Work out the finished part from the listing and answer in its coordinate system (mm). A direction names the side the tool comes from. Give positions to 0.01 mm unless a question says otherwise; leave off trailing zeros. Order: outer loops, then holes, each group sorted by start corner. A loop starts at its lowest first (then second) coordinate and runs counter-clockwise, first axis right, second up. Notation, with made-up numbers: (1, -3) -> (56, -3) arc R8 ccw to (56, 9) -> close; hole circle Ø11 at (24.5, -4.75). An arc over 180 degrees is marked (long way). Answer as CSV lines item,"result". Start each with the question number.
1. For a pull along X with two mould halves and no side action, classify faces 1 (the flat face through (0, 0, 0)), 2 (the cylindrical face through (22, 30, 5)), 3 (the flat face through (14.6, 38, -7)) as released by +X, released by -X, zero draft, split by the parting line, or undercut.
2. Find the intervals of material crossed by L1, parallel to Z at x = 24, y = 29; L2, parallel to X at y = 23.5, z = -8.5; L3, parallel to Y at x = 6, z = 3.25, in increasing order.
3. A cutting plane is placed at D-D (x = 7). Give the vertices of the cut face in (y, z), then the cut area to 3 significant figures.
4. A cutting plane is placed at B-B (x = 24.25). Give the vertices of the cut face in (y, z).
5. For faces 4 (the flat face through (20.2, 14, 0)), 5 (the flat face through (4, 38, -8.85)), 6 (the flat face through (-5, 39.6, 0)), 7 (the flat face through (-23, 3.7, 0)), 8 (the flat face through (24, 31, 0)), determine the directions among +Z, -Z, +X, -X, +Y, -Y from which every point of the face is accessible in a straight line to the end or side of a thin tool.
6. A cutting plane is placed at A-A (x = -24.25). Give the vertices of the cut face in (y, z), then the cut area to 3 significant figures.
7. A cutting plane is placed at C-C (y = 16.5). Give the vertices of the cut face in (x, z), then the cut area to 3 significant figures.
8. Flat-ended cylindrical pins translate along their axes: pin 1 (1.5 mm diameter, centred on x = 4, z = 7, fed in from +Y); pin 2 (1.7 mm diameter, centred on y = 33, z = 1.5, fed in from -X); pin 3 (1.8 mm diameter, centred on x = -24.5, z = 1, fed in from +Y). Find the tip coordinate at first contact, or state that the pin passes through.
from build123d import *

# Parameters (mm, degrees)
SKETCH1_W           = 40.4
SKETCH1_H           = 19.8
BOSS_EXTRUDE1_DEPTH = 36.7
SKETCH2_R           = 9.625
BOSS_EXTRUDE2_DEPTH = 1.7
SKETCH3_R           = 6.5
BOSS_EXTRUDE3_DEPTH = 1.2
SKETCH4_R           = 5.25
BOSS_EXTRUDE4_DEPTH = 0.5
SKETCH5_R           = 2.9
BOSS_EXTRUDE5_DEPTH = 3.8
SKETCH6_W           = 19.8
SKETCH6_H           = 2.5
BOSS_EXTRUDE6_DEPTH = 6.8
SKETCH7_R           = 2.25
CUT_EXTRUDE1_DEPTH  = 6.8
SKETCH8_W           = 7.5
SKETCH8_H           = 5
BOSS_EXTRUDE7_DEPTH = 6


with BuildPart() as part:
    # Sketch1 → Boss-Extrude1 (new body)
    with BuildSketch(Plane(origin=(0, 0, 0), x_dir=(1, 0, 0), z_dir=(0, 1, 0))):
        Rectangle(SKETCH1_W, SKETCH1_H)
    extrude(amount=BOSS_EXTRUDE1_DEPTH)

    # Sketch2 → Boss-Extrude2 (add)
    with BuildSketch(Plane(origin=(0, 36.7, 0), x_dir=(1, 0, 0), z_dir=(0, 1, 0))):
        with Locations((-10.575, 0)):
            Circle(SKETCH2_R)
        with BuildLine():
            ThreePointArc((-0.95, 0), (-2.541913742, -5.301900618), (-6.791070164, -8.85))
            Line((-6.791070164, -8.85), (14.6, -8.85))
            Line((14.6, -8.85), (14.6, -4.6))
            Line((14.6, -4.6), (14.6, 4.6))
            Line((14.6, 4.6), (14.6, 8.85))
            Line((14.6, 8.85), (-6.791070164, 8.85))
            ThreePointArc((-6.791070164, 8.85), (-2.541913742, 5.301900618), (-0.95, 0))
        make_face()
        with BuildLine():
            Line((14.6, 4.6), (14.6, -4.6))
            ThreePointArc((14.6, -4.6), (16.8, 0), (14.6, 4.6))
        make_face()
    extrude(amount=BOSS_EXTRUDE2_DEPTH)

    # Sketch3 → Boss-Extrude3 (add)
    with BuildSketch(Plane(origin=(0, 38.4, 0), x_dir=(1, 0, 0), z_dir=(0, 1, 0))):
        with Locations(Location((-10.575, 0, 0), (0, 0, 270))):
            Circle(SKETCH3_R)
    extrude(amount=BOSS_EXTRUDE3_DEPTH)

    # Sketch4 → Boss-Extrude4 (add)
    with BuildSketch(Plane(origin=(0, 39.6, 0), x_dir=(1, 0, 0), z_dir=(0, 1, 0))):
        with Locations(Location((-10.575, 0, 0), (0, 0, 270))):
            Circle(SKETCH4_R)
    extrude(amount=BOSS_EXTRUDE4_DEPTH)

    # Sketch5 → Boss-Extrude5 (add)
    with BuildSketch(Plane(origin=(0, 40.1, 0), x_dir=(1, 0, 0), z_dir=(0, 1, 0))):
        with Locations(Location((-10.575, 0, 0), (0, 0, 90))):
            Circle(SKETCH5_R)
    extrude(amount=BOSS_EXTRUDE5_DEPTH)

    # Sketch6 → Boss-Extrude6 (add)
    with BuildSketch(Plane.ZY.offset(20.2)):
        with Locations((0, 29.75)):
            Rectangle(SKETCH6_W, SKETCH6_H)
    boss_extrude6 = extrude(amount=BOSS_EXTRUDE6_DEPTH)

    # Sketch7 → Cut-Extrude1 (cut)
    with BuildSketch(Plane(origin=(0, 31, 0), x_dir=(1, 0, 0), z_dir=(0, 1, 0))):
        with Locations((-24.25, 5)):
            Circle(SKETCH7_R)
        with BuildLine():
            Line((-27, 6.25), (-27, 3.75))
            Line((-27, 3.75), (-26.120828693, 3.75))
            ThreePointArc((-26.120828693, 3.75), (-26.5, 5), (-26.120828693, 6.25))
            Line((-26.120828693, 6.25), (-27, 6.25))
        make_face()
        with Locations((-24.25, -5)):
            Circle(SKETCH7_R)
        with BuildLine():
            Line((-27, -3.75), (-27, -6.25))
            Line((-27, -6.25), (-26.120828693, -6.25))
            ThreePointArc((-26.120828693, -6.25), (-26.5, -5), (-26.120828693, -3.75))
            Line((-26.120828693, -3.75), (-27, -3.75))
        make_face()
    cut_extrude1 = extrude(amount=-CUT_EXTRUDE1_DEPTH, mode=Mode.SUBTRACT)

    # Mirror1: Boss-Extrude6, Cut-Extrude1 across plane
    add(boss_extrude6.mirror(Plane(origin=(0, 0, 0), x_dir=(0, 0, 1), z_dir=(1, 0, 0))))
    add(cut_extrude1.mirror(Plane(origin=(0, 0, 0), x_dir=(0, 0, 1), z_dir=(1, 0, 0))), mode=Mode.SUBTRACT)

    # Sketch8 → Boss-Extrude7 (add)
    with BuildSketch(Plane.ZY.offset(20.2)):
        with Locations((0, 6.2)):
            Rectangle(SKETCH8_W, SKETCH8_H)
    extrude(amount=BOSS_EXTRUDE7_DEPTH)


solid = part.part
Answer sheet:
1,face 1,"zero draft"
1,face 2,"undercut"
1,face 3,"released by +X"
2,L1,"z = -9.9 to -7.24, -2.76 to 2.76, 7.24 to 9.9"
2,L2,"x = -20.2 to 20.2"
2,L3,"y = 0 to 38.4"
3,outline,"(0, -9.9) -> (36.7, -9.9) -> (36.7, -8.85) -> (38.4, -8.85) -> (38.4, 8.85) -> (36.7, 8.85) -> (36.7, 9.9) -> (0, 9.9) -> close"
3,area,"757 mm^2"
4,outline,"(28.5, -9.9) -> (31, -9.9) -> (31, -7.25) -> (28.5, -7.25) -> close; (28.5, -2.75) -> (31, -2.75) -> (31, 2.75) -> (28.5, 2.75) -> close; (28.5, 7.25) -> (31, 7.25) -> (31, 9.9) -> (28.5, 9.9) -> close"
5,face 4,"+Z, -Z, +X, -Y"
5,face 5,"-Z, +X, +Y"
5,face 6,"+Y"
5,face 7,"+Z, -Z, -X, -Y"
5,face 8,"+Z, -Z, +X, +Y"
6,outline,"(3.7, -3.75) -> (8.7, -3.75) -> (8.7, 3.75) -> (3.7, 3.75) -> close; (28.5, -9.9) -> (31, -9.9) -> (31, -7.25) -> (28.5, -7.25) -> close; (28.5, -2.75) -> (31, -2.75) -> (31, 2.75) -> (28.5, 2.75) -> close; (28.5, 7.25) -> (31, 7.25) -> (31, 9.9) -> (28.5, 9.9) -> close"
6,area,"64.5 mm^2"
7,outline,"(-20.2, -9.9) -> (20.2, -9.9) -> (20.2, 9.9) -> (-20.2, 9.9) -> close"
7,area,"800 mm^2"
8,pin 1,"stops at y = 38.4"
8,pin 2,"stops at x = -20.2"
8,pin 3,"stops at y = 31"
